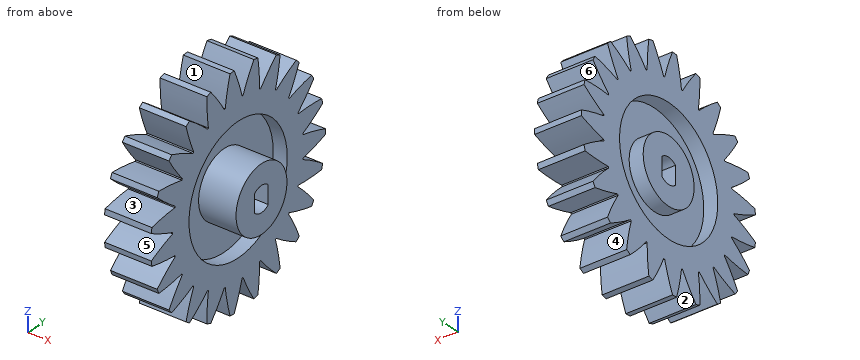
from build123d import *

# Parameters (mm, degrees)
REVOLVE_1_ANGLE          = 360
EXTRUDE_1_DEPTH          = 10
PATTERN_CIRCULAR_1_COUNT = 23
SKETCH_6_R               = 7
EXTRUDE_2_DEPTH          = 5
CUT_EXTRUDE_2_DEPTH      = 16


with BuildPart() as part:
    # 스케치3 → 회전1 (revolve, symmetric)
    with BuildSketch(Plane.XY) as revolve_1_sk:
        Polygon((-5, 18), (5, 18), (5, 13.5), (2, 13.5), (2, 7), (5, 7), (5, 0), (-5, 0), (-5, 7), (-2, 7), (-2, 13.5), (-5, 13.5), align=None)
    revolve(axis=Axis((-44.782034346, 0, 0), (1, 0, 0)), revolution_arc=REVOLVE_1_ANGLE / 2)
    revolve(revolve_1_sk.sketch, axis=Axis((-44.782034346, 0, 0), (-1, 0, 0)), revolution_arc=REVOLVE_1_ANGLE / 2)

    # 스케치4 → 보스-돌출1 (add, through all)
    with BuildSketch(Plane(origin=(5, 0, 0), x_dir=(0, 0, -1), z_dir=(1, 0, 0))):
        with BuildLine():
            ThreePointArc((0.57, 23.993230295), (0, 24), (-0.57, 23.993230295))
            Line((-0.57, 23.993230295), (-0.57, 17.990972736))
            ThreePointArc((-0.57, 17.990972736), (0.877839967, 17.978581618), (2.32, 17.849862745))
            ThreePointArc((2.32, 17.849862745), (1.565807025, 20.955959615), (0.57, 23.993230295))
        make_face()
        with BuildLine():
            Line((-0.57, 17.990972736), (-0.57, 23.993230295))
            ThreePointArc((-0.57, 23.993230295), (-1.565807025, 20.955959615), (-2.32, 17.849862745))
            ThreePointArc((-2.32, 17.849862745), (-1.446721469, 17.94176683), (-0.57, 17.990972736))
        make_face()
    extrude_1 = extrude(amount=-EXTRUDE_1_DEPTH)

    # 원형 패턴1: 보스-돌출1 ×23 about axis
    pattern_circular_1_axis = Axis((0, 0, 0), (1, 0, 0))
    for i in range(1, PATTERN_CIRCULAR_1_COUNT):
        add(extrude_1.rotate(pattern_circular_1_axis, i * 360 / PATTERN_CIRCULAR_1_COUNT))

    # 스케치6 → 보스-돌출2 (add)
    with BuildSketch(Plane(origin=(5, 0, 0), x_dir=(0, 0, -1), z_dir=(1, 0, 0))):
        Circle(SKETCH_6_R)
    extrude(amount=EXTRUDE_2_DEPTH)

    # 스케치7 → 컷-돌출2 (cut, through all)
    with BuildSketch(Plane.ZY.offset(5)):
        with BuildLine():
            Line((1.966596044, -1.85), (-1.966596044, -1.85))
            ThreePointArc((-1.966596044, -1.85), (-2.7, 0), (-1.966596044, 1.85))
            Line((-1.966596044, 1.85), (1.966596044, 1.85))
            ThreePointArc((1.966596044, 1.85), (2.7, 0), (1.966596044, -1.85))
        make_face()
    extrude(amount=-CUT_EXTRUDE_2_DEPTH, mode=Mode.SUBTRACT)


solid = part.part
Could you check a few things on this model? Use its own coordinates, in mm. Face numbers are marked on the shaded views. A direction names the side the tool comes from. Give positions to 0.01 mm unless a question says otherwise; leave off trailing zeros. Order: outer loops, then holes, each group sorted by start corner. A loop starts at its lowest first (then second) coordinate and runs counter-clockwise, first axis right, second up.
Item 1: For the marked faces 1, 2 and 3, which set-ups out of +Z, -Z, +X, -X, +Y, -Y let a thin tool reach every point of the face, with its end or its side?
Item 2: I'm going to push flat-ended pins straight in: pin 1 (1.5 mm diameter, centred on x = 7, y = 11.5, fed in from +Z); pin 2 (14.5 mm diameter, centred on y = 4.5, z = 11, fed in from +X); pin 3 (1.5 mm diameter, centred on x = -3.5, z = -14.5, fed in from +Y) (3 decimals); pin 4 (1.5 mm diameter, centred on x = 5.5, y = -8, fed in from +Z). Where does each tip first touch, or does it pass through?
Item 3: If we section it at A-A, the plane y = 19.5: Write out the boundary of the cut face in (x, z).
Item 4: If we section it at B-B, the plane x = -3: Count the separate pieces of the cut face and the enclosed holes in it, plus the area to 3 significant figures.
Item 5: If we mould it in two halves opening along Y, with no side actions, what happens to the marked faces 4, 5 and 6? For each: pulls with the +Y half, pulls with the -Y half, needs draft (parallel to the pull), parting line crosses it, or undercut.
Item 6: I need wall thicknesses on line 1 (Y direction, x = 3.55, z = 0); line 2 (Y direction, x = 3, z = -6); line 3 (Z direction, x = -2.25, y = 4). Which ranges of each line are inside material? Lowest first, please.
Item 7: If we section it at C-C, the plane y = 0: Write out the boundary of the cut face in (x, z), plus the area to 3 significant figures.
Values:
1. face 1: +Z, +X, -X
1. face 2: -Z, +X, -X
1. face 3: +X, -X, -Y
2. pin 1: passes through
2. pin 2: stops at x = 10
2. pin 3: stops at y = 15.945
2. pin 4: stops at z = 22.8
3. outline: (-5, -12.81) - (5, -12.81) - (5, -10.42) - (-5, -10.42) - close; (-5, -7.16) - (5, -7.16) - (5, -3.49) - (-5, -3.49) - close; (-5, -1.95) - (5, -1.95) - (5, 1.95) - (-5, 1.95) - close; (-5, 3.49) - (5, 3.49) - (5, 7.16) - (-5, 7.16) - close; (-5, 10.42) - (5, 10.42) - (5, 12.81) - (-5, 12.81) - close
4. separate pieces: 2
4. enclosed holes: 2
4. area: 1,000 mm2
5. face 4: undercut
5. face 5: pulls with the -Y half
5. face 6: pulls with the +Y half
6. line 1: y = -18 to -13.5, -7 to -1.85, 1.85 to 7, 13.5 to 24
6. line 2: y = -18.69 to -12.09, -3.61 to 3.61, 12.09 to 23.24
6. line 3: z = -23.08 to -12.89, -5.74 to 5.74, 12.89 to 23.08
7. outline: (-5, -21.38) - (5, -21.38) - (5, -13.5) - (2, -13.5) - (2, -7) - (10, -7) - (10, -2.7) - (-5, -2.7) - (-5, -7) - (-2, -7) - (-2, -13.5) - (-5, -13.5) - close; (-5, 2.7) - (10, 2.7) - (10, 7) - (2, 7) - (2, 13.5) - (5, 13.5) - (5, 21.38) - (-5, 21.38) - (-5, 13.5) - (-2, 13.5) - (-2, 7) - (-5, 7) - close
7. area: 339 mm2
